from build123d import *

# Parameters (mm, degrees)
SALIENTE_EXTRUIR1_DEPTH = 10.1
CROQUIS2_R              = 2.05
CORTAR_EXTRUIR1_DEPTH   = 0.5
CROQUIS3_W              = 20
CROQUIS3_H              = 1.2
CORTAR_EXTRUIR2_DEPTH   = 49.811512632
SALIENTE_EXTRUIR3_START = -7.7
SALIENTE_EXTRUIR3_DEPTH = 7.7
CROQUIS7_R              = 2.5
CORTAR_EXTRUIR4_DEPTH   = 1.5
CROQUIS8_R              = 3
SALIENTE_EXTRUIR4_DEPTH = 25
SALIENTE_EXTRUIR4_TAPER = 3


with BuildPart() as part:
    # Croquis1 → Saliente-Extruir1 (new body)
    with BuildSketch(Plane(origin=(0, 0, 0), x_dir=(1, 0, 0), z_dir=(0, 1, 0))):
        with BuildLine():
            Line((-33, -5), (33, -5))
            ThreePointArc((33, -5), (46.090169944, 0), (33, 5))
            Line((33, 5), (-33, 5))
            Line((-33, 5), (-33, -5))
        make_face()
    extrude(amount=SALIENTE_EXTRUIR1_DEPTH)

    # Croquis2 → Cortar-Extruir1 (cut)
    with BuildSketch(Plane(origin=(0, 10.1, 0), x_dir=(1, 0, 0), z_dir=(0, 1, 0))):
        with Locations(Location((38.590169944, 0, 0), (0, 0, 270))):
            Circle(CROQUIS2_R)
    extrude(amount=-CORTAR_EXTRUIR1_DEPTH, mode=Mode.SUBTRACT)

    # Croquis3 → Cortar-Extruir2 (cut, through all)
    with BuildSketch(Plane.XY.offset(5)):
        with Locations((-23, 9.5)):
            Rectangle(CROQUIS3_W, CROQUIS3_H)
    cortar_extruir2 = extrude(amount=-CORTAR_EXTRUIR2_DEPTH, mode=Mode.SUBTRACT)

    # Simetría1: Cortar-Extruir2 across plane
    add(cortar_extruir2.mirror(Plane.ZX.offset(5.05)), mode=Mode.SUBTRACT)

    # Croquis6 → Saliente-Extruir3 (add)
    with BuildSketch(Plane(origin=(0, 8.9, 0), x_dir=(1, 0, 0), z_dir=(0, 1, 0)).offset(SALIENTE_EXTRUIR3_START)):
        with BuildLine():
            Line((-33, 5), (-33, -5))
            ThreePointArc((-33, -5), (-34.754979339, -4.897304712), (-36.330136848, -5.677931145))
            ThreePointArc((-36.330136848, -5.677931145), (-43.699538391, -7.061851575), (-44.148390874, 0.422922724))
            ThreePointArc((-44.148390874, 0.422922724), (-39.122361815, 4.046630659), (-33, 5))
        make_face()
    extrude(amount=SALIENTE_EXTRUIR3_DEPTH)

    # Croquis7 → Cortar-Extruir4 (cut)
    with BuildSketch(Plane(origin=(0, 8.9, 0), x_dir=(1, 0, 0), z_dir=(0, 1, 0))):
        with Locations(Location((-40.624839531, -3.12162005, 0), (0, 0, 270))):
            Circle(CROQUIS7_R)
    cortar_extruir4 = extrude(amount=-CORTAR_EXTRUIR4_DEPTH, mode=Mode.SUBTRACT)

    # Simetría3: Cortar-Extruir4 across plane
    add(cortar_extruir4.mirror(Plane.ZX.offset(5.05)), mode=Mode.SUBTRACT)

    # Croquis8 → Saliente-Extruir4 (add)
    with BuildSketch(Plane.XZ):
        with Locations((38.590169944, 0)):
            Circle(CROQUIS8_R)
    extrude(amount=SALIENTE_EXTRUIR4_DEPTH, taper=SALIENTE_EXTRUIR4_TAPER)


solid = part.part
Geometry: final body of the model. Coordinates: model frame, mm. A direction names the side the tool comes from. Give positions to 0.01 mm unless a question says otherwise; leave off trailing zeros. Loops run counter-clockwise (first coordinate to the right, second up) from the corner with the lowest first, then second, coordinate; pieces in that order, holes last. Notation, with made-up numbers: (66, -12) - (125, -12) arc R22 cw to (125, 2) - close; hole circle Ø1 at (-38, 66.5). An arc over 180 degrees is marked (long way). Answer as CSV lines item,"result". Start each with the question number.
1. Reachability of faces 4 (the face through (-29, 8.9, 0)), 5 (the face through (40.623, 9.854, -0.267)), 6 (the face through (-29, 1.2, 0)) from +Z, -Z, +X, -X, +Y, -Y: full face, straight path, thin tool, end or side. Return the list, or none.
2. Section C-C, the plane z = -6. Return loops of the section in (x, y).
3. Section B-B, the plane y = -1. Return loops of the section in (x, z).
4. Draft query along Z for faces 1 (the face through (39, -25, 0)), 2 (the face through (-41, 7.4, 3)), 3 (the face through (0, 5, 5)). Return one class per face: released by +Z, released by -Z, zero draft, split by the parting line, or undercut.
5. Ray query, L1, parallel to X at y = 9.9, z = 0; L2, parallel to Y at x = -26.5, z = -1.75; L3, parallel to Y at x = 8, z = -3.5. Return the intervals inside material, ascending.
6. Section A-A, the plane x = -32. Return loops of the section in (y, z), plus the area to 3 significant figures.
7. Pin query (flat end, axial travel): P1, Ø1, axis at y = 0.5, z = -2.5, coming from the -X side; P2, Ø2, axis at y = 3.5, z = -4, coming from the +X side; P3, Ø2.5, axis at x = -42, z = 4, coming from the +Y side. Return the tip coordinate at first contact, or that it passes through.
Answers:
1,face 4,"+Z, -Z, -X, +Y"
1,face 5,"+Y"
1,face 6,"+Z, -Z, -X, -Y"
2,outline,"(34.09, 0) - (43.09, 0) - (43.09, 10.1) - (34.09, 10.1) - close"
3,outline,"circle Ø5.9 at (38.59, 0)"
4,face 1,"zero draft"
4,face 2,"undercut"
4,face 3,"released by +Z"
5,L1,"x = -13 to 36.54, 40.64 to 46.09"
5,L2,"y = 1.2 to 8.9"
5,L3,"y = 0 to 10.1"
6,outline,"(1.2, -5) - (8.9, -5) - (8.9, 5) - (1.2, 5) - close"
6,area,"77.0 mm2"
7,P1,"stops at x = -13"
7,P2,"stops at x = 45.46"
7,P3,"stops at y = 8.9"
